Study the drawing (mm; zero at the part's minimum x, y, z) and answer. Coordinates: 2 decimals unless noted, no trailing zeros. Loops run counter-clockwise (first coordinate to the right, second up) from the corner with the lowest first, then second, coordinate; pieces in that order, holes last. Notation, with made-up numbers: (18.5, -33.5) -> (68.5, -33.5) arc R16 cw to (68.5, -27.5) -> close; hole circle Ø5 at (75.5, 11). An arc over 180 degrees is marked (long way). Answer in a Markdown table with one row per item.
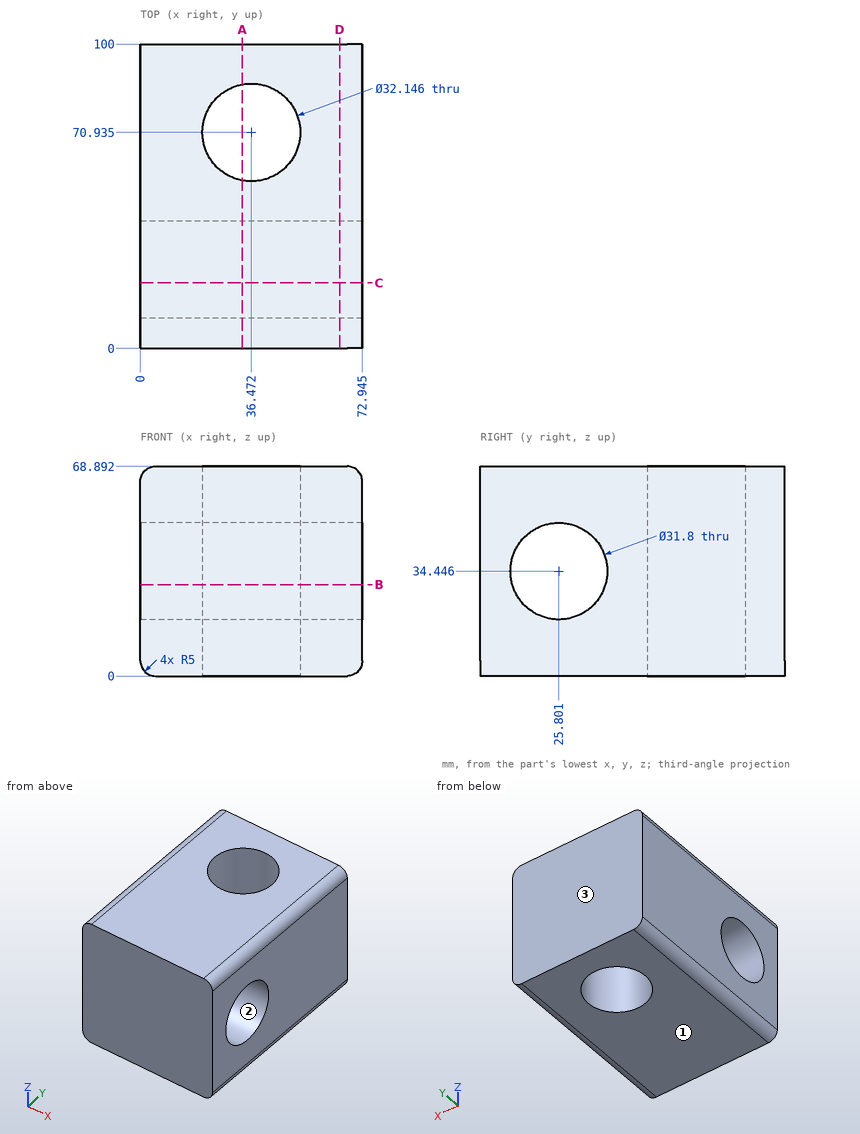
1. A cutting plane is placed at C-C on y = 21.5. Give the vertices of the cut face in (x, z) (1 decimal).
A:
| item | result |
|---|---|
| outline | (0, 5) arc R5 ccw to (5, 0) -> (67.9, 0) arc R5 ccw to (72.9, 5) -> (72.9, 19.1) -> (0, 19.1) -> close; (0, 49.8) -> (72.9, 49.8) -> (72.9, 63.9) arc R5 ccw to (67.9, 68.9) -> (5, 68.9) arc R5 ccw to (0, 63.9) -> close |
2. A cutting plane is placed at B-B on z = 30. Give the vertices of the cut face in (x, y) (1 decimal), and give its area (3 significant figures).
A:
| item | result |
|---|---|
| outline | (0, 0) -> (72.9, 0) -> (72.9, 10.5) -> (0, 10.5) -> close; (0, 41.1) -> (72.9, 41.1) -> (72.9, 100) -> (0, 100) -> close; hole circle Ø32.1 at (36.5, 70.9) |
| area | 4,260 mm2 |
3. A cutting plane is placed at D-D on x = 65.5. Give the vertices of the cut face in (y, z), and give its area (4 significant figures).
A:
| item | result |
|---|---|
| outline | (0, 0) -> (100, 0) -> (100, 68.89) -> (0, 68.89) -> close; hole circle Ø31.8 at (25.8, 34.45) |
| area | 6,095 mm2 |
4. The mould has two halves that part along Y. Classify the marked faces 1, 2 and 3: pulls with the +Y half, pulls with the -Y half, needs draft (parallel to the pull), parting line crosses it, or undercut.
A:
| item | result |
|---|---|
| face 1 | needs draft |
| face 2 | undercut |
| face 3 | pulls with the +Y half |
5. A cutting plane is placed at A-A on x = 33.5. Give the vertices of the cut face in (y, z).
A:
| item | result |
|---|---|
| outline | (0, 0) -> (55.14, 0) -> (55.14, 68.89) -> (0, 68.89) -> close; (86.73, 0) -> (100, 0) -> (100, 68.89) -> (86.73, 68.89) -> close; hole circle Ø31.8 at (25.8, 34.45) |
6. Find the intervals of material crossed by probe 1 along Y at (x, z) = (37.5, 29) (1 decimal); probe 2 along Y at (x, z) = (28.5, 30.5); probe 3 along X at (y, z) = (60, 10) (1 decimal), in increasing order.
A:
| item | result |
|---|---|
| probe 1 | y = 0 to 10.9, 40.7 to 54.9, 87 to 100 |
| probe 2 | y = 0 to 10.4, 41.2 to 56.98, 84.89 to 100 |
| probe 3 | x = 0 to 24.7, 48.3 to 72.9 |
